Verification items for the finished model (mm, model axes). A direction names the side the tool comes from. Round coordinates to 2 decimals unless told otherwise and drop trailing zeros. Write each loop counter-clockwise with the first axis right and the second up, starting at its lowest first coordinate (ties: lowest second). Pieces come first, ordered by that corner, then holes. Notation, with made-up numbers: (28, 7) -> (53, 7) arc R29 cw to (53, 38) -> close; hole circle Ø3 at (43.5, 11.25). An arc over 180 degrees is marked (long way). Answer as a JSON object with one key per item and string values. Group by question number.
(1) Scan lines: L1, parallel to Z at x = 12, y = -3.25; L2, parallel to Z at x = 2.75, y = -10.75; L3, parallel to X at y = -15, z = 3. Record each from-to range of solid material in increasing order. Write a range as from..to.
(2) Sectioned sample at B-B on z = -2.5. Record the cut outline in (x, y), and give its area (3 significant figures).
(3) Sectioned sample at D-D on y = -16. Record the cut outline in (x, z).
(4) Set-up check for faces 4 (the face through (12.5, -0.5, -3.3)), 5 (the face through (6, -9, 12.6)), 6 (the face through (13, -9, 6)): record each of +Z, -Z, +X, -X, +Y, -Y from which the full face is reachable in a straight line by a thin tool's end or side.
(5) Sectioned sample at C-C on x = 3.5. Record the cut outline in (y, z), and give its area (3 significant figures).
(6) Gauge pin test, flat ends, axial feed: pin 1 Ø3.5 at (x, y) = (6, -5) entering from -Z; pin 2 Ø5 at (x, y) = (3, -13.5) entering from -Z. Record the tip position at first contact, or that the pin passes through.
(7) Draft check along Z on faces 1 (the face through (12.5, -7.5, -3.3)), 2 (the face through (6, -9, 14)), 3 (the face through (12.6, -9, 7)). Enter one of: released by +Z, released by -Z, zero draft, split by the parting line, or undercut.
(8) Sectioned sample at A-A on y = -3.25. Record the cut outline in (x, z).
```python
from build123d import *

# Parameters (mm, degrees)
F0_W     = 13
F0_H     = 14
F1_DEPTH = 17.5
F2_W     = 12.2
F2_H     = 13.2
F2_W_2   = 11.2
F2_H_2   = 1.5
F2_H_3   = 3.4
F3_DEPTH = 17
F4_W     = 13
F4_H     = 8
F5_DEPTH = 1.5
F6_W     = 0.5
F6_H     = 1
F7_DEPTH = 3.7
F8_R     = 0.5


with BuildPart() as f1:
    # F0 (on Front) → F1 (new body)
    with BuildSketch(Plane.XZ):
        with Locations((6.5, 7)):
            Rectangle(F0_W, F0_H)
    extrude(amount=F1_DEPTH)

    # F2 (on face) → F3 (cut)
    with BuildSketch(Plane.XZ.offset(17.5)):
        with Locations((6.5, 7)):
            Rectangle(F2_W, F2_H)
        with Locations((6.5, 3.55)):
            Rectangle(F2_W_2, F2_H_2, mode=Mode.SUBTRACT)
        with Locations((6.5, 7)):
            Rectangle(F2_W_2, F2_H_3, mode=Mode.SUBTRACT)
        with Locations((6.5, 11.85)):
            Rectangle(F2_W_2, F2_H_2, mode=Mode.SUBTRACT)
    extrude(amount=-F3_DEPTH, mode=Mode.SUBTRACT)

    # F4 (on face) → F5 (join)
    with BuildSketch(Plane(origin=(0, 0, 0), x_dir=(1, 0, 0), z_dir=(0, 0, -1))):
        with Locations((6.5, 4)):
            Rectangle(F4_W, F4_H)
    extrude(amount=F5_DEPTH)

    # F6 (on face) → F7 (join)
    with BuildSketch(Plane(origin=(0, 0, -1.5), x_dir=(1, 0, 0), z_dir=(0, 0, -1))):
        with Locations((0.25, 7.5)):
            Rectangle(F6_W, F6_H)
        with Locations((0.25, 0.5)):
            Rectangle(F6_W, F6_H)
        with Locations((12.75, 7.5)):
            Rectangle(F6_W, F6_H)
        with Locations((12.75, 0.5)):
            Rectangle(F6_W, F6_H)
    extrude(amount=F7_DEPTH)

    # F8
    f8_edges = [f1.edges().sort_by_distance(p)[0] for p in [
        (13, -8.75, 14),
        (6.5, 0, 14),
        (0, -8.75, 14),
    ]]
    fillet(f8_edges, radius=F8_R)


solid = f1.part
```
Computed values:
{
 "1": {"L1": "-1.5..0.4, 2.8..4.3, 5.3..8.7, 11.1..12.6, 13.6..14", "L2": "0..0.4, 2.8..4.3, 5.3..8.7, 11.1..12.6, 13.6..14", "L3": "0..0.4, 0.9..12.1, 12.6..13"},
 "2": {"outline": "(0, -8) -> (0.5, -8) -> (0.5, -7) -> (0, -7) -> close; (0, -1) -> (0.5, -1) -> (0.5, 0) -> (0, 0) -> close; (12.5, -8) -> (13, -8) -> (13, -7) -> (12.5, -7) -> close; (12.5, -1) -> (13, -1) -> (13, 0) -> (12.5, 0) -> close", "area": "2.00 mm2"},
 "3": {"outline": "(0, 0) -> (13, 0) -> (13, 13.5) arc R0.5 ccw to (12.5, 14) -> (0.5, 14) arc R0.5 ccw to (0, 13.5) -> close; (0.9, 2.8) -> (12.1, 2.8) -> (12.1, 4.3) -> (0.9, 4.3) -> close; (0.9, 5.3) -> (12.1, 5.3) -> (12.1, 8.7) -> (0.9, 8.7) -> close; (0.9, 11.1) -> (12.1, 11.1) -> (12.1, 12.6) -> (0.9, 12.6) -> close; hole (0.4, 0.4) -> (12.6, 0.4) -> (12.6, 13.6) -> (0.4, 13.6) -> close"},
 "4": {"face 4": "-Z, +Y, -Y", "face 5": "-Y", "face 6": "+Z, -Z, +X, +Y, -Y"},
 "5": {"outline": "(-17.5, 0) -> (-8, 0) -> (-8, -1.5) -> (0, -1.5) -> (0, 13.5) arc R0.5 ccw to (-0.5, 14) -> (-17.5, 14) -> (-17.5, 13.6) -> (-0.5, 13.6) -> (-0.5, 12.6) -> (-17.5, 12.6) -> (-17.5, 11.1) -> (-0.5, 11.1) -> (-0.5, 8.7) -> (-17.5, 8.7) -> (-17.5, 5.3) -> (-0.5, 5.3) -> (-0.5, 4.3) -> (-17.5, 4.3) -> (-17.5, 2.8) -> (-0.5, 2.8) -> (-0.5, 0.4) -> (-17.5, 0.4) -> close", "area": "141 mm2"},
 "6": {"pin 1": "z = -1.5", "pin 2": "z = 0"},
 "7": {"face 1": "zero draft", "face 2": "released by +Z", "face 3": "undercut"},
 "8": {"outline": "(0, -1.5) -> (13, -1.5) -> (13, 13.5) arc R0.5 ccw to (12.5, 14) -> (0.5, 14) arc R0.5 ccw to (0, 13.5) -> close; (0.9, 2.8) -> (12.1, 2.8) -> (12.1, 4.3) -> (0.9, 4.3) -> close; (0.9, 5.3) -> (12.1, 5.3) -> (12.1, 8.7) -> (0.9, 8.7) -> close; (0.9, 11.1) -> (12.1, 11.1) -> (12.1, 12.6) -> (0.9, 12.6) -> close; hole (0.4, 0.4) -> (12.6, 0.4) -> (12.6, 13.6) -> (0.4, 13.6) -> close"}
}
